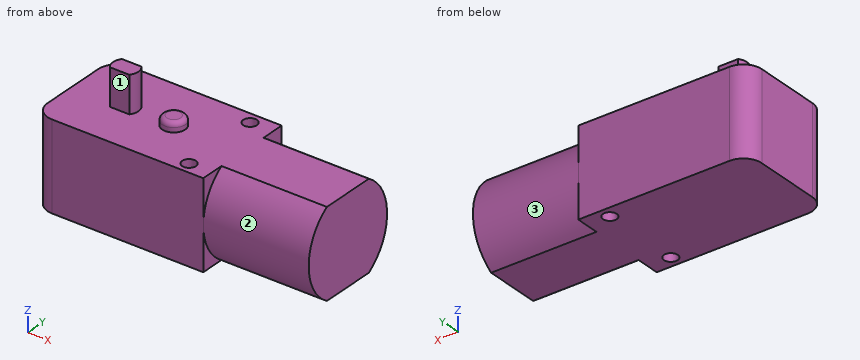
from build123d import *

# Parameters (mm, degrees)
BOSS_EXTRUDE1_DEPTH = 19
BOSS_EXTRUDE2_DEPTH = 23
BOSS_EXTRUDE3_DEPTH = 8
SKETCH4_R           = 2.5
BOSS_EXTRUDE4_DEPTH = 2
FILLET1_R           = 1
SKETCH5_R           = 1.5
CUT_EXTRUDE1_DEPTH  = 48.008642822


with BuildPart() as part:
    # Sketch1 → Boss-Extrude1 (new body)
    with BuildSketch(Plane.XY):
        with BuildLine():
            Line((-14.5, 11.25), (18.5, 11.25))
            Line((18.5, 11.25), (18.5, -11.25))
            Line((18.5, -11.25), (-14.5, -11.25))
            ThreePointArc((-14.5, -11.25), (-17.328427125, -10.078427125), (-18.5, -7.25))
            Line((-18.5, -7.25), (-18.5, 7.25))
            ThreePointArc((-18.5, 7.25), (-17.328427125, 10.078427125), (-14.5, 11.25))
        make_face()
    extrude(amount=BOSS_EXTRUDE1_DEPTH)

    # Sketch2 → Boss-Extrude2 (add)
    with BuildSketch(Plane(origin=(18.5, 0, 0), x_dir=(0, 0, -1), z_dir=(1, 0, 0))):
        with BuildLine():
            Line((-19, 6.025985397), (-19, -6.025985397))
            ThreePointArc((-19, -6.025985397), (-9.5, -11.25), (0, -6.025985397))
            Line((0, -6.025985397), (0, 6.025985397))
            ThreePointArc((0, 6.025985397), (-9.5, 11.25), (-19, 6.025985397))
        make_face()
    extrude(amount=BOSS_EXTRUDE2_DEPTH)

    # Sketch3 → Boss-Extrude3 (add)
    with BuildSketch(Plane.XY.offset(19)):
        with BuildLine():
            Line((-9.121320344, 1.75), (-4.878679656, 1.75))
            ThreePointArc((-4.878679656, 1.75), (-4.25, 0), (-4.878679656, -1.75))
            Line((-4.878679656, -1.75), (-9.121320344, -1.75))
            ThreePointArc((-9.121320344, -1.75), (-9.75, 0), (-9.121320344, 1.75))
        make_face()
    extrude(amount=BOSS_EXTRUDE3_DEPTH)

    # Sketch4 → Boss-Extrude4 (add)
    with BuildSketch(Plane.XY.offset(19)):
        with Locations((3.5, 0)):
            Circle(SKETCH4_R)
    extrude(amount=BOSS_EXTRUDE4_DEPTH)

    # Fillet1
    fillet1_edges = [part.edges().sort_by_distance(p)[0] for p in [
        (1, 0, 21),
    ]]
    fillet(fillet1_edges, radius=FILLET1_R)

    # Sketch5 → Cut-Extrude1 (cut, through all)
    with BuildSketch(Plane.XY.offset(19)):
        with Locations((13.5, 8.75)):
            Circle(SKETCH5_R)
        with Locations((13.5, -8.75)):
            Circle(SKETCH5_R)
    extrude(amount=-CUT_EXTRUDE1_DEPTH, mode=Mode.SUBTRACT)


solid = part.part
Geometry: final body of the model. Coordinates: model frame, mm. Face numbers are marked on the shaded views. A direction names the side the tool comes from. Round coordinates to 2 decimals unless told otherwise and drop trailing zeros. Order: outer loops, then holes, each group sorted by start corner. A loop starts at its lowest first (then second) coordinate and runs counter-clockwise, first axis right, second up. Notation, with made-up numbers: (25.25, -37.75) - (76.25, -37.75) arc R23 ccw to (76.25, 1.25) - close; hole circle Ø3 at (-31, -7.5). An arc over 180 degrees is marked (long way). Write each question's results on one line, items separated by ' | '.
Item 1: Section A-A, the plane x = 13.5. Return the cut outline in (y, z), and give its area (4 significant figures).
Completed:
outline: (-11.25, 0) - (-10.25, 0) - (-10.25, 19) - (-11.25, 19) - close; (-7.25, 0) - (7.25, 0) - (7.25, 19) - (-7.25, 19) - close; (10.25, 0) - (11.25, 0) - (11.25, 19) - (10.25, 19) - close | area: 313.5 mm^2
Item 2: Section B-B, the plane y = 0. Return the cut outline in (x, z).
Completed:
outline: (-18.5, 0) - (41.5, 0) - (41.5, 19) - (6, 19) - (6, 20) arc R1 ccw to (5, 21) - (2, 21) arc R1 ccw to (1, 20) - (1, 19) - (-4.25, 19) - (-4.25, 27) - (-9.75, 27) - (-9.75, 19) - (-18.5, 19) - close
Item 3: Section C-C, the plane z = 14.5. Return the cut outline in (x, y), and give its area (3 significant figures).
Completed:
outline: (-18.5, -7.25) arc R4 ccw to (-14.5, -11.25) - (18.5, -11.25) - (18.5, -10.08) - (41.5, -10.08) - (41.5, 10.08) - (18.5, 10.08) - (18.5, 11.25) - (-14.5, 11.25) arc R4 ccw to (-18.5, 7.25) - close; hole circle Ø3 at (13.5, -8.75); hole circle Ø3 at (13.5, 8.75) | area: 1,280 mm^2
Item 4: Section D-D, the plane y = -8.75. Return the cut outline in (x, z), and give its area (3 significant figures).
Completed:
outline: (-18.21, 0) - (12, 0) - (12, 19) - (-18.21, 19) - close; (15, 0) - (18.5, 0) - (18.5, 2.43) - (41.5, 2.43) - (41.5, 16.57) - (18.5, 16.57) - (18.5, 19) - (15, 19) - close | area: 966 mm^2
Item 5: First-contact query: pin 1 Ø4.5 at (x, z) = (-6, 23) entering from -Y; pin 2 Ø5 at (y, z) = (8.5, 11.5) entering from -X; pin 3 Ø2.5 at (x, y) = (13.5, -8.75) entering from +Z; pin 4 Ø11 at (x, y) = (18, -3) entering from +Z. Flat tips, straight axial feed; report the tip coordinate or a pass-through.
Completed:
pin 1: y = -1.75 | pin 2: x = -18.5 | pin 3: through | pin 4: z = 19
Item 6: Reachability of the marked faces 1, 2 and 3 from +Z, -Z, +X, -X, +Y, -Y: full face, straight path, thin tool, end or side. Return the list, or none.
Completed:
face 1: +Z, -X, -Y | face 2: +X, -Y | face 3: +X, +Y
Item 7: Material intervals for line 1 along Y through (x, z) = (13.5, 12.25); line 2 along Z through (x, y) = (7, -10.25); line 3 along X through (y, z) = (-10, 11.25), sorted ascending. Write a range as [from, to].
Completed:
line 1: [-11.25, -10.25], [-7.25, 7.25], [10.25, 11.25] | line 2: [0, 19] | line 3: [-17.4, 12.67], [14.33, 41.5]
